Verification items for the finished model (mm, model axes). A direction names the side the tool comes from. Give positions to 0.01 mm unless a question says otherwise; leave off trailing zeros.
from build123d import *

# Parameters (mm, degrees)
BOSS_EXTRUDE1_DEPTH  = 1.5875
M4_CLEARANCE_HOLE1_D = 4.5
BOSS_EXTRUDE2_DEPTH  = 3.175
M3_CLEARANCE_HOLE1_D = 3.4
FILLET1_R            = 3.5
SKETCH8_R            = 4
CUT_EXTRUDE1_DEPTH   = 4.1750001


with BuildPart() as part:
    # Sketch2 → Boss-Extrude1 (new body, symmetric)
    with BuildSketch(Plane.XY):
        with BuildLine():
            add(Edge.make_bspline(
                [(-24.777431429, -6.350183234), (-24.299810251, -5.902972393), (-23.32289496, -5.01651393), (-22.058866471, -3.944003435), (-21.276036232, -3.316259916), (-20.98344634, -3.086723573)],
                knots=[0, 0, 0, 0, 0.03125, 0.0625, 0.081068463, 0.081068463, 0.081068463, 0.081068463], degree=3))
            Line((-24.777431429, -6.350183234), (-21.36, -10))
            add(Edge.make_bspline(
                [(-21.36, -10), (-20.09052587, -8.81135381), (-18.821051739, -7.728673603), (-17.551577609, -6.751959378)],
                knots=[0, 0, 0, 0, 0.089148464, 0.089148464, 0.089148464, 0.089148464], degree=3))
            Line((-17.551577609, -6.751959378), (-20.98344634, -3.086723573))
        make_face()
        with BuildLine():
            Line((-21.36, -10), (-24.777431429, -6.350183234))
            ThreePointArc((-24.777431429, -6.350183234), (-26.357299125, -9.8356788), (-25.009816701, -13.417431499))
            ThreePointArc((-25.009816701, -13.417431499), (-21.5243212, -14.997299125), (-17.942568571, -13.649816766))
            Line((-17.942568571, -13.649816766), (-21.36, -10))
        make_face()
        with BuildLine():
            ThreePointArc((-25.009816701, -13.417431499), (-26.357299125, -9.8356788), (-24.777431429, -6.350183234))
            add(Edge.make_bspline(
                [(-24.777431429, -6.350183234), (-24.299810251, -5.902972393), (-23.32289496, -5.01651393), (-22.058866471, -3.944003435), (-21.276036232, -3.316259916), (-20.98344634, -3.086723573)],
                knots=[0, 0, 0, 0, 0.03125, 0.0625, 0.081068463, 0.081068463, 0.081068463, 0.081068463], degree=3))
            Line((-20.98344634, -3.086723573), (-21.127614663, -2.932751805))
            Line((-21.127614663, -2.932751805), (-23.519816663, -0.377880068))
            ThreePointArc((-23.519816663, -0.377880068), (-30.587064859, -0.145494731), (-30.819450196, -7.212742926))
            Line((-30.819450196, -7.212742926), (-28.427248195, -9.767614663))
            Line((-28.427248195, -9.767614663), (-25.009816701, -13.417431499))
        make_face()
        with BuildLine():
            add(Edge.make_bspline(
                [(-21.36, -10), (-20.09052587, -8.81135381), (-18.821051739, -7.728673603), (-17.551577609, -6.751959378)],
                knots=[0, 0, 0, 0, 0.089148464, 0.089148464, 0.089148464, 0.089148464], degree=3))
            Line((-21.36, -10), (-17.942568571, -13.649816766))
            add(Edge.make_bspline(
                [(-17.942568571, -13.649816766), (-17.543072686, -13.275756949), (-16.7212792, -12.530114496), (-15.44829951, -11.450473224), (-14.582019434, -10.770813046), (-14.116024052, -10.421130577)],
                knots=[0, 0, 0, 0, 0.03125, 0.0625, 0.099339971, 0.099339971, 0.099339971, 0.099339971], degree=3))
            Line((-14.116024052, -10.421130577), (-14.292751805, -10.232385337))
            Line((-14.292751805, -10.232385337), (-17.551577609, -6.751959378))
        make_face()
        with BuildLine():
            ThreePointArc((-17.942568571, -13.649816766), (-21.5243212, -14.997299125), (-25.009816701, -13.417431499))
            Line((-25.009816701, -13.417431499), (-21.592385337, -17.067248195))
            Line((-21.592385337, -17.067248195), (-19.200183337, -19.622119932))
            ThreePointArc((-19.200183337, -19.622119932), (-12.132935141, -19.854505269), (-11.900549804, -12.787257074))
            Line((-11.900549804, -12.787257074), (-14.116024052, -10.421130577))
            add(Edge.make_bspline(
                [(-17.942568571, -13.649816766), (-17.543072686, -13.275756949), (-16.7212792, -12.530114496), (-15.44829951, -11.450473224), (-14.582019434, -10.770813046), (-14.116024052, -10.421130577)],
                knots=[0, 0, 0, 0, 0.03125, 0.0625, 0.099339971, 0.099339971, 0.099339971, 0.099339971], degree=3))
        make_face()
        with BuildLine():
            add(Edge.make_bspline(
                [(-20.98344634, -3.086723573), (-20.291201445, -2.543658465), (-18.603117827, -1.28817338), (-15.885096675, 0.462779531), (-11.785009924, 2.624744664), (-6.509375137, 4.48808894), (0, 5.25595553), (6.509375137, 4.48808894), (11.785009924, 2.624744664), (15.885096675, 0.462779531), (18.901874802, -1.480633029), (21.37388106, -3.362802893), (23.32289496, -5.01651393), (24.299810251, -5.902972393), (24.777431429, -6.350183234)],
                knots=[0.081068463, 0.081068463, 0.081068463, 0.081068463, 0.125, 0.1875, 0.25, 0.375, 0.5, 0.625, 0.75, 0.8125, 0.875, 0.9375, 0.96875, 1, 1, 1, 1], degree=3))
            Line((-20.98344634, -3.086723573), (-17.551577609, -6.751959378))
            Line((-17.551577609, -6.751959378), (-14.292751805, -10.232385337))
            Line((-14.292751805, -10.232385337), (-14.116024052, -10.421130577))
            add(Edge.make_bspline(
                [(-14.116024052, -10.421130577), (-13.791445759, -10.177567349), (-12.680801028, -9.370838959), (-10.815202086, -8.171392792), (-7.794818062, -6.582915934), (-4.170679183, -5.321481205), (0, -4.839259398), (4.170679183, -5.321481205), (7.794818062, -6.582915934), (10.815202086, -8.171392792), (13.136984474, -9.664132159), (15.119482265, -11.171596294), (16.7212792, -12.530114496), (17.543072686, -13.275756949), (17.942568571, -13.649816766)],
                knots=[0.099339971, 0.099339971, 0.099339971, 0.099339971, 0.125, 0.1875, 0.25, 0.375, 0.5, 0.625, 0.75, 0.8125, 0.875, 0.9375, 0.96875, 1, 1, 1, 1], degree=3))
            ThreePointArc((17.942568571, -13.649816766), (25.009816766, -13.417431429), (24.777431429, -6.350183234))
        make_face()
    extrude(amount=BOSS_EXTRUDE1_DEPTH, both=True)

    # M4 Clearance Hole1 (through all)
    with Locations(Plane.XY.offset(1.5875)):
        with Locations((-21.359999999, -9.999999999), (0, 0), (-15.550366571, -16.204688503), (-27.169633429, -3.795311497)):
            Hole(M4_CLEARANCE_HOLE1_D / 2)

    # Sketch5 → Boss-Extrude2 (add)
    with BuildSketch(Plane(origin=(0, 0, -1.5875), x_dir=(-1, 0, 0), z_dir=(0, 0, -1))):
        with BuildLine():
            ThreePointArc((-23.201229183, -22.868950039), (-17.11, -26.460179221), (-13.518770817, -20.368950039))
            Line((-13.518770817, -20.368950039), (-16.518770817, -8.75))
            ThreePointArc((-16.518770817, -8.75), (-22.61, -5.158770817), (-26.201229183, -11.25))
            Line((-26.201229183, -11.25), (-23.201229183, -22.868950039))
        make_face()
    extrude(amount=-BOSS_EXTRUDE2_DEPTH)

    # M3 Clearance Hole1 (through all)
    with Locations(Plane(origin=(0, 0, -1.5875), x_dir=(-1, 0, 0), z_dir=(0, 0, -1))):
        with Locations((-18.36, -21.618950039)):
            Hole(M3_CLEARANCE_HOLE1_D / 2)

    # Fillet1
    fillet1_edges = [part.edges().sort_by_distance(p)[0] for p in [
        (15.75315909, -11.715201468, -0.79375),
        (-20.98344634, -3.086723573, -0.79375),
        (-14.116024052, -10.421130577, 0.79375),
    ]]
    fillet(fillet1_edges, radius=FILLET1_R)

    # Sketch8 → Cut-Extrude1 (cut, through all)
    with BuildSketch(Plane(origin=(0, 0, -1.5875), x_dir=(-1, 0, 0), z_dir=(0, 0, -1))):
        with Locations((-21.36, -10)):
            Circle(SKETCH8_R)
    extrude(amount=-CUT_EXTRUDE1_DEPTH, mode=Mode.SUBTRACT)


solid = part.part
Item 1: Scan lines: line 1 along Y through (x, z) = (0, 0.8); line 2 along X through (y, z) = (-18, 1.25); line 3 along Y through (x, z) = (18.36, 0.9). Record each from-to range of solid material in increasing order.
Answer key:
line 1: y = -5 to -2.25, 2.25 to 5
line 2: x = -20.72 to -16.91, -14.19 to -10.88, 14.13 to 24.46
line 3: y = -26.62 to -23.32, -19.92 to -12.65, -7.35 to -1.16
Item 2: Set-up check for faces 1 (the face through (24.72, -16.98, -0.02)), 2 (the face through (14.34, -17.19, -0.02)): record each of +Z, -Z, +X, -X, +Y, -Y from which the full face is reachable in a straight line by a thin tool's end or side.
Answer key:
face 1: +Z, -Z, +X, -Y
face 2: +Z, -Z
Item 3: Sectioned sample at A-A on x = 18.36. State how many separate pieces and enclosed holes the cut face has, then the cut area to 3 significant figures.
Answer key:
separate pieces: 3
enclosed holes: 0
area: 53.2 mm2
Item 4: Release check for a two-part mould opening along X. For faces 3 (the face through (-2, -3, 1.588)), 4 (the face through (26.17, -8.64, 0.02)), 5 (the face through (-13.303, -16.106, -0.022)) record: released by +X, released by -X, zero draft, split by the parting line, or undercut.
Answer key:
face 3: zero draft
face 4: released by +X
face 5: undercut
Item 5: Depth check by flat-ended pin: pin 1 (5 mm diameter, centred on x = -21.36, y = -10, fed in from -Z). Enter the tip coordinate at first touch or a pass-through.
Answer key:
pin 1: stops at z = -1.59
